Can you work these out from the drawing? Everything is in mm from the part's minimum corner. A direction names the side the tool comes from. Round coordinates to 2 decimals unless told otherwise and drop trailing zeros. Loops run counter-clockwise (first coordinate to the right, second up) from the corner with the lowest first, then second, coordinate; pieces in that order, holes last. Notation, with made-up numbers: (40.5, -28.75) - (92.5, -28.75) arc R26 cw to (92.5, -10.75) - close; hole circle Ø1 at (76.5, -2.5). An arc over 180 degrees is marked (long way). Answer as CSV lines item,"result". Start each with the question number.
1) Which directions (+Z, -Z, +X, -X, +Y, -Y) give clear straight access to the entire face, cutting with the end or side of a thin tool? Please do the marked faces 4 and 5.
2) Please list where these lines run through material, in increasing order: line 1 along X through (y, z) = (22.5, 58.5) (1 decimal); line 2 along X through (y, z) = (5, 49); line 3 along Z through (x, y) = (153.5, 7.5) (1 decimal).
3) We'd pull the mould along X, two halves only. Please class the marked faces 1, 2 and 3: pulls with the +X half, pulls with the -X half, needs draft (parallel to the pull), parting line crosses it, or undercut.
4) I'm going to push flat-ended pins straight in: pin 1 Ø1.5 at (y, z) = (14, 53.5) entering from +X; pin 2 Ø12 at (x, y) = (154.5, 9) entering from +Z. Where does each tip first touch, or does it pass through?
5) Suppose I cut it at C-C, the plane x = 142. Write out the boundary of the cut face in (y, z), then the cut area to 3 significant figures.
6) Suppose I cut it at B-B, the plane y = 21. Write out the boundary of the cut face in (x, z) (1 decimal).
7) Suppose I cut it at A-A, the plane z = 47.5. Write out the boundary of the cut face in (x, y), then the cut area to 3 significant figures.
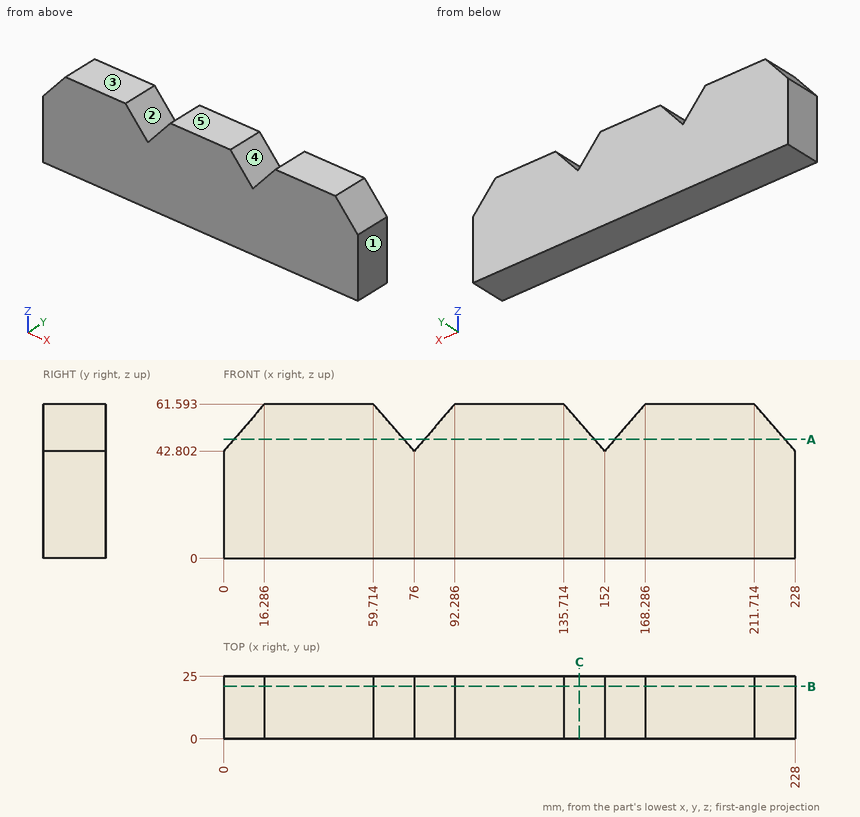
Filled sheet:
1,face 4,"+Z, +Y, -Y"
1,face 5,"+Z, +X, -X, +Y, -Y"
2,line 1,"13.6 to 62.4, 89.6 to 138.4, 165.6 to 214.4"
2,line 2,"5.37 to 70.63, 81.37 to 146.63, 157.37 to 222.63"
2,line 3,"0 to 44.5"
3,face 1,"pulls with the +X half"
3,face 2,"undercut"
3,face 3,"needs draft"
4,pin 1,"x = 219.38"
4,pin 2,"z = 52.61"
5,outline,"(0, 0) - (25, 0) - (25, 54.34) - (0, 54.34) - close"
5,area,"1,360 mm²"
6,outline,"(0, 0) - (228, 0) - (228, 42.8) - (211.7, 61.6) - (168.3, 61.6) - (152, 42.8) - (135.7, 61.6) - (92.3, 61.6) - (76, 42.8) - (59.7, 61.6) - (16.3, 61.6) - (0, 42.8) - close"
7,outline,"(4.07, 0) - (71.93, 0) - (71.93, 25) - (4.07, 25) - close; (80.07, 0) - (147.93, 0) - (147.93, 25) - (80.07, 25) - close; (156.07, 0) - (223.93, 0) - (223.93, 25) - (156.07, 25) - close"
7,area,"5,090 mm²"
